Drawing for the job (mm, zero at the part's lowest x, y, z). Round coordinates to 2 decimals unless told otherwise and drop trailing zeros. Write each loop counter-clockwise with the first axis right and the second up, starting at its lowest first coordinate (ties: lowest second). Pieces come first, ordered by that corner, then holes.
Item 1: Drop flat-ended pins along their axis: pin 1 Ø3 at (x, y) = (4.5, 17) entering from +Z; pin 2 Ø6 at (y, z) = (19.5, 16.5) entering from +X; pin 3 Ø1.5 at (y, z) = (16, 13) entering from -X. Give the stop position or say it passes through.
Item 2: Band-saw the part on A-A, the plane x = 14.25. Write the cut outline in (y, z).
Item 3: Wall check: probe 1 along Y at (x, z) = (21.86, 6.6) (3 decimals); probe 2 along Z at (x, y) = (11.75, 23.25); probe 3 along X at (y, z) = (13.5, 3.75) (3 decimals). Give the ranges that are in metal, low to high.
Item 4: Band-saw the part on B-B, the plane z = 5. Write the cut outline in (x, y) (3 decimals).
Item 5: Band-saw the part on D-D, the plane x = 21.86. Write the cut outline in (y, z) (3 decimals).
Item 6: Band-saw the part on C-C, the plane z = 17. Write the cut outline in (x, y) (3 decimals), then the cut area to 3 significant figures.
Item 7: Mould opens along Y. For the marked faces 1, 2 and 3 say: +Y half, -Y half, draft (parallel to the pull), parting line (faces both ways), or undercut.
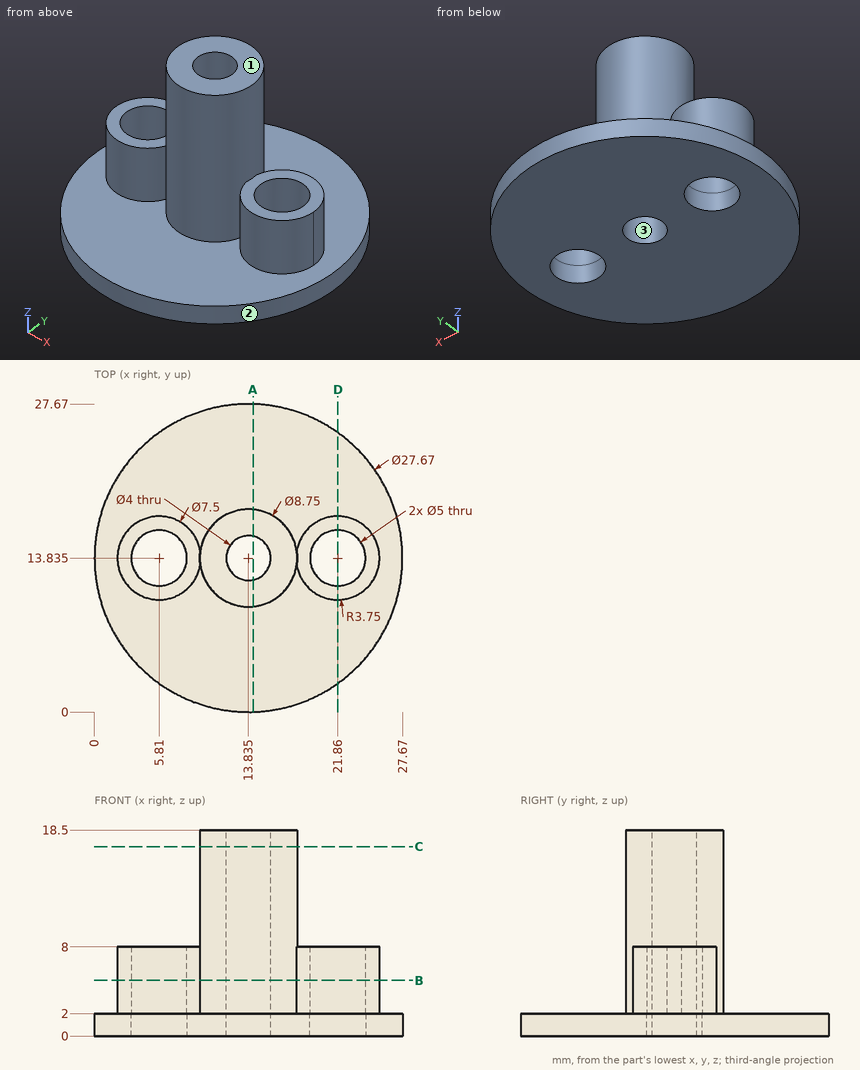
Results:
1. pin 1: stops at z = 8
1. pin 2: stops at x = 17.3
1. pin 3: stops at x = 9.7
2. outline: (0.01, 0) - (11.88, 0) - (11.88, 18.5) - (9.48, 18.5) - (9.48, 2) - (0.01, 2) - close; (15.79, 0) - (27.66, 0) - (27.66, 2) - (18.19, 2) - (18.19, 18.5) - (15.79, 18.5) - close
3. probe 1: y = 10.085 to 11.335, 16.335 to 17.585
3. probe 2: z = 0 to 2
3. probe 3: x = 2.075 to 3.333, 8.287 to 11.863, 15.807 to 19.383, 24.337 to 25.595
4. outline: (9.506, 13.202) arc R4.375 ccw to (18.164, 13.202) arc R3.75 ccw (long way) to (18.164, 14.468) arc R4.375 ccw to (9.506, 14.468) arc R3.75 ccw (long way) to start; hole circle Ø5 at (5.81, 13.835); hole circle Ø4 at (13.835, 13.835); hole circle Ø5 at (21.86, 13.835)
5. outline: (2.565, 0) - (11.335, 0) - (11.335, 8) - (10.085, 8) - (10.085, 2) - (2.565, 2) - close; (16.335, 0) - (25.105, 0) - (25.105, 2) - (17.585, 2) - (17.585, 8) - (16.335, 8) - close
6. outline: circle Ø8.75 at (13.835, 13.835); hole circle Ø4 at (13.835, 13.835)
6. area: 47.6 mm2
7. face 1: draft
7. face 2: parting line
7. face 3: undercut
